```python
from build123d import *

# Parameters (mm, degrees)
F1_DEPTH = 76.2
F3_DEPTH = 25
F5_DEPTH = 25


with BuildPart() as f1:
    # F0 (on Top) → F1 (new body)
    with BuildSketch(Plane.XY):
        with BuildLine():
            Line((-29.137894, 0), (-16.437894, 0))
            ThreePointArc((-16.437894, 0), (-2.614066, 4.412701), (11.562106, 1.313299))
            Line((11.562106, 1.313299), (24.262106, 1.313299))
            ThreePointArc((24.262106, 1.313299), (-2.67384, 10.250454), (-29.137894, 0))
        make_face()
    extrude(amount=F1_DEPTH)

    # F2 (on Front) → F3 (cut)
    with BuildSketch(Plane.XZ):
        Polygon((25.847133, 41.631106), (24.586304, 78.813426), (-30.959083, 78.813426), align=None)
    extrude(amount=-F3_DEPTH, mode=Mode.SUBTRACT)

    # F4 (on Front) → F5 (cut)
    with BuildSketch(Plane.XZ):
        Polygon((-34.645859, -3.21119), (-3.547264, -3.21119), (-3.547264, 18.966397), (-19.190293, 34.029976), (-34.645859, 34.029976), align=None)
    extrude(amount=-F5_DEPTH, mode=Mode.SUBTRACT)


solid = f1.part
```
The listing builds one solid part. Answer for the finished solid, in the listing's coordinates (mm). A direction names the side the tool comes from. Give positions to 0.01 mm unless a question says otherwise; leave off trailing zeros. Loops run counter-clockwise (first coordinate to the right, second up) from the corner with the lowest first, then second, coordinate; pieces in that order, holes last. Notation, with made-up numbers: M 42,41 L 57,41 A23 ccw 57,58 Z; hole C -30,11.25 d10. An arc over 180 degrees is marked long. One line per item, written item: value.
1. Section C-C on x = -4.5 is taken. Determine the outline of the cut face in (y, z).
Found:
outline: M 4.26,19.88 L 10.17,19.88 L 10.17,61.49 L 4.26,61.49 Z
2. Section A-A on y = 5.5 is taken. Determine the outline of the cut face in (x, z).
Found:
outline: M -21.06,34.03 L -19.19,34.03 L -3.55,18.97 L -3.55,0 L 17.78,0 L 17.78,46.91 L -21.06,72.33 Z
3. For faces 1 (the face through (18, 1.313, 25)), 2 (the face through (-2.27, 10.26, 37.57)), 3 (the face through (-23, 2, 34.03)), determine the directions among +Z, -Z, +X, -X, +Y, -Y from which every point of the face is accessible in a straight line to the end or side of a thin tool.
Found:
face 1: +Z, -Z, +X, -Y
face 2: +Z, -Z, +Y
face 3: -Z, -X, +Y, -Y
4. Each of these flat-tipped pins is pushed along its axis until it touches: P1, Ø1.5, axis at x = -17.5, z = 61, coming from the +Y side; P2, Ø8, axis at x = -4, z = 62.5, coming from the -Y side; P3, Ø3, axis at x = 10, z = 53.5, coming from the -Y side. Where does it stop, or does it pass through?
Found:
P1: y = 7.45
P2: y = 3.63
P3: y = 2.06
5. Find the intervals of material crossed by probe 1 along X at (y, z) = (1.5, 51); probe 2 along X at (y, z) = (6.5, 41); probe 3 along Z at (x, y) = (-15, 5.25), in increasing order.
Found:
probe 1: -27.31 to -13.8, 11.19 to 11.53
probe 2: -19.01 to 15.73
probe 3: 29.99 to 68.37
6. Section B-B on z = 11.5 is taken. Determine the outline of the cut face in (x, y), plus the area to 3 significant figures.
Found:
outline: M -3.55,4.35 A28 cw 11.56,1.31 L 24.26,1.31 A41.96 ccw -3.55,10.22 Z
area: 141 mm^2
